Input: part model. Units: mm. Frame: model coordinates. A direction names the side the tool comes from. Coordinates: 2 decimals unless noted, no trailing zeros. Loops run counter-clockwise (first coordinate to the right, second up) from the corner with the lowest first, then second, coordinate; pieces in that order, holes last. Notation, with made-up numbers: (21, 65.5) -> (72, 65.5) arc R28 cw to (72, 94.5) -> close; hole circle Ø3 at (64, 1). An arc over 180 degrees is marked (long way). Answer as a JSON object with one key per item and string values.
from build123d import *

# Parameters (mm, degrees)
CROQUIS1_R              = 2
SALIENTE_EXTRUIR1_DEPTH = 3
CHAFL_N1_SIZE           = 3


with BuildPart() as part:
    # Croquis1 → Saliente-Extruir1 (new body)
    with BuildSketch(Plane(origin=(0, 0, 0), x_dir=(1, 0, 0), z_dir=(0, 1, 0))):
        Polygon((-15, 11.288045039), (-15, 30), (15, 30), (15, 11.288045039), (5.54714751, -10), (-34.833084075, -10), (-34.833084075, 0), (-20.012401302, 0), align=None)
        with Locations(Location((-29.833084075, -5, 0), (0, 0, 270))):
            Circle(CROQUIS1_R, mode=Mode.SUBTRACT)
        with BuildLine():
            Line((-10, 17.5), (10, 17.5))
            ThreePointArc((10, 17.5), (12.5, 20), (10, 22.5))
            Line((10, 22.5), (-10, 22.5))
            ThreePointArc((-10, 22.5), (-12.5, 20), (-10, 17.5))
        make_face(mode=Mode.SUBTRACT)
    extrude(amount=SALIENTE_EXTRUIR1_DEPTH)

    # Chaflán1
    chafl_n1_edges = [part.edges().sort_by_distance(p)[0] for p in [
        (-34.833084075, 1.5, 10),
        (-34.833084075, 1.5, 0),
        (-15, 1.5, -30),
        (15, 1.5, -30),
    ]]
    chamfer(chafl_n1_edges, length=CHAFL_N1_SIZE)


solid = part.part
1. Section query A-A (x = 1). Return loops of the section in (y, z), plus the area to 3 significant figures.
Reply:
{"outline": "(0, -30) -> (3, -30) -> (3, -22.5) -> (0, -22.5) -> close; (0, -17.5) -> (3, -17.5) -> (3, 10) -> (0, 10) -> close", "area": "105 mm2"}
2. Pin query (flat end, axial travel): P1, Ø1, axis at x = -14.5, z = 0.5, coming from the -Y side; P2, Ø0.9, axis at y = 2, z = -22, coming from the -X side. Return the tip coordinate at first contact, or that it passes through.
Reply:
{"P1": "stops at y = 0", "P2": "stops at x = -15"}
3. Section query B-B (z = -20). Return loops of the section in (x, y), plus the area to 3 significant figures.
Reply:
{"outline": "(-15, 0) -> (-12.5, 0) -> (-12.5, 3) -> (-15, 3) -> close; (12.5, 0) -> (15, 0) -> (15, 3) -> (12.5, 3) -> close", "area": "15.0 mm2"}
4. Section query C-C (y = 1.8). Return loops of the section in (x, z).
Reply:
{"outline": "(-34.83, 3) -> (-31.83, 0) -> (-20.01, 0) -> (-15, -11.29) -> (-15, -27) -> (-12, -30) -> (12, -30) -> (15, -27) -> (15, -11.29) -> (5.55, 10) -> (-31.83, 10) -> (-34.83, 7) -> close; hole circle Ø4 at (-29.83, 5); hole (-10, -22.5) -> (10, -22.5) arc R2.5 ccw to (10, -17.5) -> (-10, -17.5) arc R2.5 ccw to start"}
5. Section query D-D (x = -21). Return loops of the section in (y, z).
Reply:
{"outline": "(0, 0) -> (3, 0) -> (3, 10) -> (0, 10) -> close"}
6. Mould query, pull axis Z, two halves, no side actions, for faces 4 (the face through (14, 1, -28)), 5 (the face through (15, 1, -19)), 6 (the face through (12.5, 1.5, -19.9)). Classes: pulls with the +Z half, pulls with the -Z half, needs draft (parallel to the pull), parting line crosses it, or undercut.
Reply:
{"face 4": "pulls with the -Z half", "face 5": "needs draft", "face 6": "undercut"}
7. Line query: line 1 along Z through (x, y) = (-1.5, 0.95); line 2 along Z through (x, y) = (-29, 0.2); line 3 along X through (y, z) = (2.65, -27). Output: solid intervals per line, ascending.
Reply:
{"line 1": "z = -30 to -22.5, -17.5 to 10", "line 2": "z = 0 to 3.18, 6.82 to 10", "line 3": "x = -15 to 15"}
8. Access query for faces 1 (the face through (-15, 1, -19)), 2 (the face through (-4, 3, -6)), 3 (the face through (0, 1, -17.5)). Directions: +Z, -Z, +X, -X, +Y, -Y. A direction counts if a zero-diameter tool reaches every point of the face in a straight line with its end or side. Return the directions, or none.
Reply:
{"face 1": "-Z, -X, +Y, -Y", "face 2": "+Z, -Z, +X, -X, +Y", "face 3": "+Y, -Y"}
